```python
from build123d import *

# Parameters (mm, degrees)
BASENUTSKE_R  = 2.5527
BASENUT_DEPTH = 5.7404


with BuildPart() as part:
    # BaseNutSke → BaseNut (new body)
    with BuildSketch(Plane.XY):
        Polygon((5.55625, 3.207902433), (5.55625, -3.207902433), (0, -6.415804866), (-5.55625, -3.207902433), (-5.55625, 3.207902433), (0, 6.415804866), align=None)
        Circle(BASENUTSKE_R, mode=Mode.SUBTRACT)
    extrude(amount=-BASENUT_DEPTH)

    # Sketch3 → Double-Chamfer (revolve, cut)
    with BuildSketch(Plane(origin=(0, 0, 0), x_dir=(0, 0, -1), z_dir=(1, 0, 0))):
        Polygon((5.7404, 5.55625), (5.1054, 6.415804866), (5.1054, 19.115804866), (18.4404, 19.115804866), (18.4404, 5.55625), align=None)
        Polygon((0.635, 19.115804866), (-12.7, 19.115804866), (-12.7, 5.55625), (0, 5.55625), (0.635, 6.415804866), align=None)
    revolve(axis=Axis((0, 0, 0), (0, 0, -1)), mode=Mode.SUBTRACT)

    # Sketch5 → EndChamfer (revolve, cut)
    with BuildSketch(Plane(origin=(0, 0, 0), x_dir=(0, 0, -1), z_dir=(1, 0, 0))):
        Polygon((5.715, 3.175), (5.235686934, 2.49047), (5.7658, 2.49047), (5.7658, 3.175), align=None)
        Polygon((-0.0508, 3.175), (0, 3.175), (0.479313066, 2.49047), (-0.0508, 2.49047), align=None)
    revolve(axis=Axis((0, 0, -25.037505729), (0, 0, -1)), mode=Mode.SUBTRACT)


solid = part.part
```
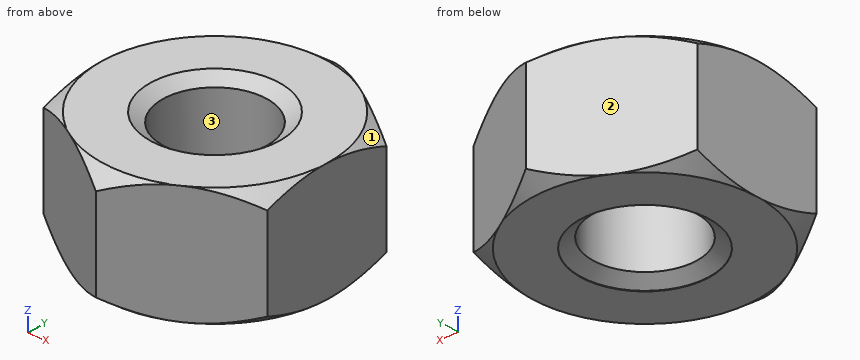
Source: CAD feature listing. Evaluate the final solid. Frame: model axes, mm. Face numbers are marked on the shaded views. Give positions to 0.01 mm unless a question says otherwise; leave off trailing zeros. Write each loop counter-clockwise with the first axis right and the second up, starting at its lowest first coordinate (ties: lowest second). Pieces come first, ordered by that corner, then holes.
1. Section query A-A (z = -3.2). Return the cut outline in (x, y), then the cut area to 3 significant figures.
2. First-contact query: pin 1 (4.5 mm diameter, centred on x = 0, y = 0, fed in from -Z); pin 2 (1.5 mm diameter, centred on x = 0.5, z = -2.5, fed in from +Y); pin 3 (1 mm diameter, centred on x = 1, z = -5, fed in from -Y); pin 4 (1.5 mm diameter, centred on x = -2.5, z = -4.5, fed in from +Y). Flat tips, straight axial feed; report the tip coordinate or a pass-through.
3. Material intervals for line 1 along X through (y, z) = (0, -2.15); line 2 along Y through (x, z) = (-0.25, -1.15); line 3 along Y through (x, z) = (0, -5.65), sorted ascending.
4. Pull-direction query (X, two-part tool) for the marked faces 1, 2 and 3; classes: +X half, -X half, draft (parallel to the pull), parting line (faces both ways), or undercut.
Output values:
1. outline: (-5.56, -3.21) - (0, -6.42) - (5.56, -3.21) - (5.56, 3.21) - (0, 6.42) - (-5.56, 3.21) - close; hole circle Ø5.11 at (0, 0)
1. area: 86.5 mm2
2. pin 1: passes through
2. pin 2: stops at y = 6.42
2. pin 3: stops at y = -6.13
2. pin 4: stops at y = 5.41
3. line 1: x = -5.56 to -2.55, 2.55 to 5.56
3. line 2: y = -6.27 to -2.54, 2.54 to 6.27
3. line 3: y = -5.68 to -3.08, 3.08 to 5.68
4. face 1: +X half
4. face 2: -X half
4. face 3: undercut
